```python
from build123d import *

# Parameters (mm, degrees)
SKETCH1_W           = 9.53
SKETCH1_H           = 9.53
BOSS_EXTRUDE1_DEPTH = 5.08
SKETCH2_R           = 3.81
BOSS_EXTRUDE2_DEPTH = 0.1
SKETCH3_R           = 3.175
BOSS_EXTRUDE3_DEPTH = 0.51
SKETCH4_R           = 1.5875
BOSS_EXTRUDE4_DEPTH = 5.08


with BuildPart() as part:
    # Sketch1 → Boss-Extrude1 (new body)
    with BuildSketch(Plane.XY):
        with Locations((4.765, 4.765)):
            Rectangle(SKETCH1_W, SKETCH1_H)
    extrude(amount=BOSS_EXTRUDE1_DEPTH)

    # Sketch2 → Boss-Extrude2 (add)
    with BuildSketch(Plane.XY.offset(5.08)):
        with Locations(Location((4.765, 4.765, 0), (0, 0, 180))):
            Circle(SKETCH2_R)
    extrude(amount=BOSS_EXTRUDE2_DEPTH)

    # Sketch3 → Boss-Extrude3 (add)
    with BuildSketch(Plane.XY.offset(5.18)):
        with Locations((4.765, 4.765)):
            Circle(SKETCH3_R)
    extrude(amount=BOSS_EXTRUDE3_DEPTH)

    # Sketch4 → Boss-Extrude4 (add)
    with BuildSketch(Plane.XY.offset(5.69)):
        with Locations((4.765, 4.765)):
            Circle(SKETCH4_R)
    extrude(amount=BOSS_EXTRUDE4_DEPTH)


solid = part.part
```
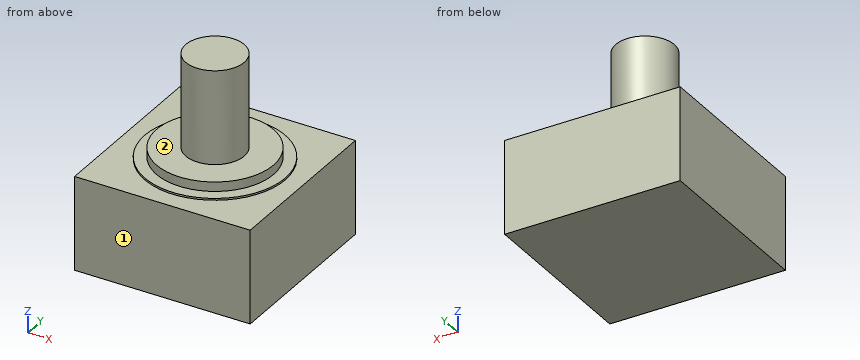
Source: CAD feature listing. Evaluate the final solid. Frame: model axes, mm. Face numbers are marked on the shaded views. A direction names the side the tool comes from. Round coordinates to 2 decimals unless told otherwise and drop trailing zeros. Loops run counter-clockwise (first coordinate to the right, second up) from the corner with the lowest first, then second, coordinate; pieces in that order, holes last.
(1) Section query D-D (y = 2). Output: boundary loops of the cut face in (x, z), and give its area (3 significant figures).
From the geometry:
outline: (0, 0) - (9.53, 0) - (9.53, 5.08) - (7.39, 5.08) - (7.39, 5.18) - (6.33, 5.18) - (6.33, 5.69) - (3.2, 5.69) - (3.2, 5.18) - (2.14, 5.18) - (2.14, 5.08) - (0, 5.08) - close
area: 50.5 mm2
(2) Contact query for flat-ended pins moving along their axis: pin 1 Ø1 at (x, y) = (7.5, 7) entering from +Z; pin 2 Ø5 at (x, z) = (8.5, 9) entering from -Y; pin 3 Ø2 at (x, y) = (8.5, 1.5) entering from +Z. Output: stop coordinate, or through.
From the geometry:
pin 1: stops at z = 5.69
pin 2: stops at y = 3.77
pin 3: stops at z = 5.08
(3) Material intervals for probe 1 along Z at (x, y) = (2.5, 3.75); probe 2 along Z at (x, y) = (9, 6.5); probe 3 along X at (y, z) = (4.75, 5.75), sorted ascending.
From the geometry:
probe 1: z = 0 to 5.69
probe 2: z = 0 to 5.08
probe 3: x = 3.18 to 6.35
(4) Access query for the marked faces 1 and 2. Directions: +Z, -Z, +X, -X, +Y, -Y. A direction counts if a zero-diameter tool reaches every point of the face in a straight line with its end or side. Return the directions, or none.
From the geometry:
face 1: +Z, -Z, +X, -X, -Y
face 2: +Z
(5) Section query B-B (x = 7.75). Output: boundary loops of the cut face in (y, z), and give its area (3 significant figures).
From the geometry:
outline: (0, 0) - (9.53, 0) - (9.53, 5.08) - (7.13, 5.08) - (7.13, 5.18) - (5.85, 5.18) - (5.85, 5.69) - (3.68, 5.69) - (3.68, 5.18) - (2.4, 5.18) - (2.4, 5.08) - (0, 5.08) - close
area: 50.0 mm2
(6) Section query C-C (z = 10.25). Output: boundary loops of the cut face in (x, y) (1 decimal), and give its area (3 significant figures).
From the geometry:
outline: circle Ø3.2 at (4.8, 4.8)
area: 7.92 mm2
(7) Section query A-A (y = 4). Output: boundary loops of the cut face in (x, z), and give its area (3 significant figures).
From the geometry:
outline: (0, 0) - (9.53, 0) - (9.53, 5.08) - (8.5, 5.08) - (8.5, 5.18) - (7.85, 5.18) - (7.85, 5.69) - (6.16, 5.69) - (6.16, 10.77) - (3.37, 10.77) - (3.37, 5.69) - (1.68, 5.69) - (1.68, 5.18) - (1.03, 5.18) - (1.03, 5.08) - (0, 5.08) - close
area: 66.4 mm2
